Autodesk Inventor part; units mm, degrees
ref_plane "YZ Plane" through (0, 0, 0) normal (1, 0, 0) x (0, 1, 0)
ref_plane "XZ Plane" through (0, 0, 0) normal (0, 1, 0) x (-1, 0, 0)
ref_plane "XY Plane" through (0, 0, 0) normal (0, 0, 1) x (1, 0, 0)
sketch "Sketch1" plane through (0, 0, 0) normal (0, 1, 0) x (-1, 0, 0)
  arc A0 (3.1129, -2) -> (0, 3.7) centre (0, 0) ccw
  line L0 (3.1129, -2) -> (3.7086, -2.8032)
  arc A1 (3.7086, -2.8032) -> (0.5, 4.6218) centre (0, 0) ccw
  line L1 (0, 10) -> (0.5, 10)
  line L2 (0.5, 10) -> (0.5, 4.6218)
  line L3 (0, 3.7) -> (0, 10)
  arc A2 (0, 3.7) -> (-3.1129, -2) centre (0, 0) ccw
  line L4 (-3.1129, -2) -> (-3.7086, -2.8032)
  arc A3 (-0.5, 4.6218) -> (-3.7086, -2.8032) centre (0, 0) ccw
  line L5 (0, 10) -> (-0.5, 10)
  line L6 (-0.5, 10) -> (-0.5, 4.6218)
  dimension "d0" = 10
  dimension "d1" = 7.4
  dimension "d3" = 1
  dimension "d4" = 0.5
extrude "Extrusion1" add sketch "Sketch1" along normal blind 3
properties part number "Microphone holder"
Geometry check sheet. Reference: the model listing, model coordinates, mm. A direction names the side the tool comes from. Round coordinates to 2 decimals unless told otherwise and drop trailing zeros. Loops run counter-clockwise (first coordinate to the right, second up) from the corner with the lowest first, then second, coordinate; pieces in that order, holes last. Notation, with made-up numbers: (11, 2.5) - (37, 2.5) arc R21 ccw to (37, 7.5) - close; hole circle Ø9 at (-25.75, -26). An arc over 180 degrees is marked (long way). One line per question, with ' | ' between items. Start each with the question number.
1. Cross-section at B-B on z = 3. Record the cut outline in (x, y), then the cut area to 3 significant figures.
2. Cross-section at C-C on x = 3.25. Record the cut outline in (y, z).
3. Tool access check on faces 1 (the face through (3.41, 1.48, -2.4)), 2 (the face through (0.5, 1, 7)), 3 (the face through (-3.22, 1.48, 1.82)). Record the directions out of +Z, -Z, +X, -X, +Y, -Y that give a thin tool (end or side, any length) a straight path to the whole face; none if there is none.
4. Depth check by flat-ended pin: pin 1 (1.5 mm diameter, centred on y = 1.5, z = 4.5, fed in from +X); pin 2 (3 mm diameter, centred on x = -1.5, z = 5.5, fed in from -Y); pin 3 (0.9 mm diameter, centred on y = 1, z = 6, fed in from -X); pin 4 (1.5 mm diameter, centred on x = 3.5, y = 1, fed in from +Z). Enter the tip coordinate at first touch or a pass-through.
5. Draft check along X on faces 4 (the face through (0, 3, 4)), 5 (the face through (-0.5, 1, 7)), 6 (the face through (3.274, 1.479, 1.725)). Enter one of: released by +X, released by -X, zero draft, split by the parting line, or undercut.
6. Scan lines: line 1 (X direction, y = 1.7, z = 7); line 2 (X direction, y = 2.55, z = 0.5); line 3 (X direction, y = 0.85, z = 2.75). Record each from-to range of solid material in increasing order. Write a range as [from, to].
7. Cross-section at A-A on y = 1.85. Record the cut outline in (x, z).
8. Cross-section at D-D on z = 9. Record the cut outline in (x, y).
Taken from the geometry:
1) outline: (-3.55, 0) - (-2.17, 0) - (-2.17, 3) - (-3.55, 3) - close; (2.17, 0) - (3.55, 0) - (3.55, 3) - (2.17, 3) - close | area: 8.31 mm²
2) outline: (0, -2.18) - (3, -2.18) - (3, -1.77) - (0, -1.77) - close; (0, 1.77) - (3, 1.77) - (3, 3.32) - (0, 3.32) - close
3) face 1: -Z, +Y, -Y | face 2: +Z, +X, +Y, -Y | face 3: +Y, -Y
4) pin 1: x = 2.75 | pin 2: y = 0 | pin 3: x = -0.5 | pin 4: z = 3.75
5) face 4: zero draft | face 5: released by -X | face 6: undercut
6) line 1: [-0.5, 0.5] | line 2: [-4.62, -3.67], [3.67, 4.62] | line 3: [-3.75, -2.48], [2.48, 3.75]
7) outline: (-3.71, -2.8) - (-3.11, -2) arc R3.7 cw to (0, 3.7) arc R3.7 cw to (3.11, -2) - (3.71, -2.8) arc R4.65 ccw to (0.5, 4.62) - (0.5, 10) - (-0.5, 10) - (-0.5, 4.62) arc R4.65 ccw to start
8) outline: (-0.5, 0) - (0.5, 0) - (0.5, 3) - (-0.5, 3) - close
